from build123d import *

# Parameters (mm, degrees)
SKETCH1_R           = 12.5
BOSS_EXTRUDE1_DEPTH = 112
SKETCH2_R           = 10
BOSS_EXTRUDE2_DEPTH = 9
BOSS_EXTRUDE3_START = 9
SKETCH3_R           = 10
BOSS_EXTRUDE3_DEPTH = 9
SKETCH4_W           = 13
SKETCH4_H           = 6.35
CUT_EXTRUDE1_DEPTH  = 2.38125
BOSS_EXTRUDE5_START = 70
SKETCH6_R           = 10
BOSS_EXTRUDE5_DEPTH = 70


with BuildPart() as part:
    # Sketch1 → Boss-Extrude1 (new body)
    with BuildSketch(Plane.XY):
        Circle(SKETCH1_R)
    extrude(amount=BOSS_EXTRUDE1_DEPTH)

    # Sketch2 → Boss-Extrude2 (add)
    with BuildSketch(Plane.XY.offset(112)):
        Circle(SKETCH2_R)
    extrude(amount=BOSS_EXTRUDE2_DEPTH)

    # Sketch3 → Boss-Extrude3 (add)
    with BuildSketch(Plane(origin=(0, 0, 0), x_dir=(-1, 0, 0), z_dir=(0, 0, -1)).offset(BOSS_EXTRUDE3_START)):
        with Locations(Location((0, 0, 0), (0, 0, 180))):
            Circle(SKETCH3_R)
    extrude(amount=-BOSS_EXTRUDE3_DEPTH)

    # Sketch4 → Cut-Extrude1 (cut)
    with BuildSketch(Plane(origin=(12.5, 0, 0), x_dir=(0, 0, -1), z_dir=(1, 0, 0))):
        with Locations((-56, 0)):
            Rectangle(SKETCH4_W, SKETCH4_H)
    extrude(amount=-CUT_EXTRUDE1_DEPTH, mode=Mode.SUBTRACT)

    # Sketch6 → Boss-Extrude5 (add)
    with BuildSketch(Plane(origin=(0, 0, -9), x_dir=(-1, 0, 0), z_dir=(0, 0, -1)).offset(BOSS_EXTRUDE5_START)):
        with Locations(Location((0, 0, 0), (0, 0, 180))):
            Circle(SKETCH6_R)
    extrude(amount=-BOSS_EXTRUDE5_DEPTH)


solid = part.part
Input: part model. Units: mm. Frame: model coordinates. A direction names the side the tool comes from. Give positions to 0.01 mm unless a question says otherwise; leave off trailing zeros. Write each loop counter-clockwise with the first axis right and the second up, starting at its lowest first coordinate (ties: lowest second). Pieces come first, ordered by that corner, then holes. Notation, with made-up numbers: (-40, 60) -> (-32, 60) arc R13 ccw to (-32, 74) -> close; hole circle Ø8 at (86.5, 64.25). An arc over 180 degrees is marked (long way). Use one line per item in the form item = value. Start each with the question number.
1) Section query A-A on x = 0. Return the cut outline in (y, z), then the cut area to 3 significant figures.
2) Pin query (flat end, axial travel): pin 1 (1.2 mm diameter, centred on x = 11.5, y = 1, fed in from +Z); pin 2 (4 mm diameter, centred on x = 6.5, z = 21, fed in from -Y); pin 3 (10 mm diameter, centred on y = -2.5, z = -10, fed in from +X). Return the tip coordinate at first contact, or that it passes through.
3) Section query D-D on y = -8. Return the cut outline in (x, z).
4) Ray query, probe 1 along Z at (x, y) = (10.5, -2.75); probe 2 along Z at (x, y) = (-7.75, 7); probe 3 along Y at (x, z) = (-0.75, 68). Return the intervals inside material, ascending. Write a range as from..to.
5) Set-up query: faces 4 (the flat face through (0, 0, 121)), 5 (the cylindrical face through (-2.17, -9.76, 116.44)). Return all of +Z, -Z, +X, -X, +Y, -Y with unobstructed straight access to the full face (end or side cutting, diameter ignored); none if empty.
6) Section query B-B on y = 0. Return the cut outline in (x, z), then the cut area to 3 significant figures.
7) Section query C-C on z = 81.5. Return the cut outline in (x, y).
8) Draft query along Y for faces 1 (the flat face through (10.119, 0, 56)), 2 (the cylindrical face through (-10, 0, -40)), 3 (the flat face through (-0.1, 10.2, 0)). Return one class per face: pulls with the +Y half, pulls with the -Y half, needs draft (parallel to the pull), parting line crosses it, or undercut.
Outcome:
q1.outline = (-12.5, 0) -> (-10, 0) -> (-10, -79) -> (10, -79) -> (10, 0) -> (12.5, 0) -> (12.5, 112) -> (10, 112) -> (10, 121) -> (-10, 121) -> (-10, 112) -> (-12.5, 112) -> close
q1.area = 4,560 mm^2
q2.pin_1 = 112
q2.pin_2 = -11.66
q2.pin_3 = 10
q3.outline = (-9.6, 0) -> (-6, 0) -> (-6, -79) -> (6, -79) -> (6, 0) -> (9.6, 0) -> (9.6, 112) -> (6, 112) -> (6, 121) -> (-6, 121) -> (-6, 112) -> (-9.6, 112) -> close
q4.probe_1 = 0..49.5, 62.5..112
q4.probe_2 = 0..112
q4.probe_3 = -12.48..12.48
q5.face_4 = +Z, +X, -X, +Y, -Y
q5.face_5 = +Z
q6.outline = (-12.5, 0) -> (-10, 0) -> (-10, -79) -> (10, -79) -> (10, 0) -> (12.5, 0) -> (12.5, 49.5) -> (10.12, 49.5) -> (10.12, 62.5) -> (12.5, 62.5) -> (12.5, 112) -> (10, 112) -> (10, 121) -> (-10, 121) -> (-10, 112) -> (-12.5, 112) -> close
q6.area = 4,530 mm^2
q7.outline = circle Ø25 at (0, 0)
q8.face_1 = undercut
q8.face_2 = parting line crosses it
q8.face_3 = needs draft
